The model under review builds one solid part; all positions refer to its coordinate system, in mm. Coordinates: 2 decimals unless noted, no trailing zeros. Loops run counter-clockwise (first coordinate to the right, second up) from the corner with the lowest first, then second, coordinate; pieces in that order, holes last. Notation, with made-up numbers: M -2,39 L 26,39 A21 ccw 26,55 Z; hole C 44,40.5 d4. An arc over 180 degrees is marked long. One line per item, written item: value.
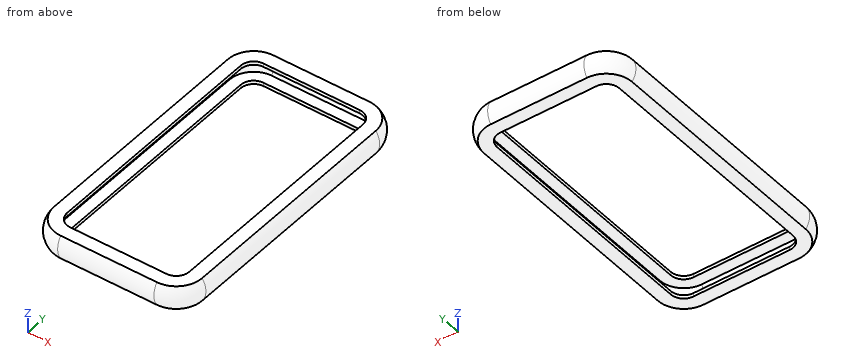
```python
from build123d import *

# Parameters (mm, degrees)
F1_DEPTH  = 5
F3_DEPTH  = 49
F5_DEPTH  = 20.5
F15_DEPTH = 1.5
F17_T     = 1.5


# Not quite as in the source:
# - a shell that OpenCascade refuses in one call is made with other operations: the cavity is built on its own and cut out


with BuildPart() as f1:
    # F0 (on Top) → F1 (new body, symmetric)
    with BuildSketch(Plane.XY):
        with BuildLine():
            Line((31.5, -49), (31.5, 49))
            ThreePointArc((31.5, 49), (28.2781745931, 56.7781745931), (20.5, 60))
            Line((20.5, 60), (-20.5, 60))
            ThreePointArc((-20.5, 60), (-28.2781745931, 56.7781745931), (-31.5, 49))
            Line((-31.5, 49), (-31.5, -49))
            ThreePointArc((-31.5, -49), (-28.2781745931, -56.7781745931), (-20.5, -60))
            Line((-20.5, -60), (20.5, -60))
            ThreePointArc((20.5, -60), (28.2781745931, -56.7781745931), (31.5, -49))
        make_face()
        with BuildLine():
            ThreePointArc((-29.5, 49), (-26.8639610307, 55.3639610307), (-20.5, 58))
            Line((-20.5, 58), (20.5, 58))
            ThreePointArc((20.5, 58), (26.8639610307, 55.3639610307), (29.5, 49))
            Line((29.5, 49), (29.5, -49))
            ThreePointArc((29.5, -49), (26.8639610307, -55.3639610307), (20.5, -58))
            Line((20.5, -58), (-20.5, -58))
            ThreePointArc((-20.5, -58), (-26.8639610307, -55.3639610307), (-29.5, -49))
            Line((-29.5, -49), (-29.5, 49))
        make_face(mode=Mode.SUBTRACT)
    extrude(amount=F1_DEPTH, both=True)

    # F2 (on Front) → F3 (join, symmetric)
    with BuildSketch(Plane.XZ):
        with BuildLine():
            Line((-31.5, -5), (-31.5, 5))
            ThreePointArc((-31.5, 5), (-33.1261364576, 0), (-31.5, -5))
        make_face()
        with BuildLine():
            ThreePointArc((31.5, -5), (33.1261364576, 0), (31.5, 5))
            Line((31.5, 5), (31.5, -5))
        make_face()
    extrude(amount=F3_DEPTH, both=True)

    # F4 (on Right) → F5 (join, symmetric)
    with BuildSketch(Plane.YZ):
        with BuildLine():
            ThreePointArc((60, -5), (61.6261364576, 0), (60, 5))
            Line((60, 5), (60, -5))
        make_face()
        with BuildLine():
            Line((-60, -5), (-60, 5))
            ThreePointArc((-60, 5), (-61.6261364576, 0), (-60, -5))
        make_face()
    extrude(amount=F5_DEPTH, both=True)

    # F7: sweep along a path in F0
    with BuildLine(Plane.XY) as f7_path:
        ThreePointArc((-20.5, 62), (-29.6923881554, 58.1923881554), (-33.5, 49))
    # F6 (on face) → F7 (sweep)
    with BuildSketch(Plane(origin=(-20.5, 0, 0), x_dir=(0, -1, 0), z_dir=(-1, 0, 0))):
        with BuildLine():
            ThreePointArc((-60, 5), (-61.6261364576, 0), (-60, -5))
            Line((-60, -5), (-60, 5))
        make_face()
    sweep(path=f7_path.line)

    # F9: sweep along a path in F0
    with BuildLine(Plane.XY) as f9_path:
        ThreePointArc((33.5, 49), (29.6923881554, 58.1923881554), (20.5, 62))
    # F8 (on face) → F9 (sweep)
    with BuildSketch(Plane.YZ.offset(20.5)):
        with BuildLine():
            Line((60, 5), (60, -5))
            ThreePointArc((60, -5), (61.6261364576, 0), (60, 5))
        make_face()
    sweep(path=f9_path.line)

    # F11: sweep along a path in F0
    with BuildLine(Plane.XY) as f11_path:
        ThreePointArc((20.5, -62), (29.6923881554, -58.1923881554), (33.5, -49))
    # F10 (on face) → F11 (sweep)
    with BuildSketch(Plane.YZ.offset(20.5)):
        with BuildLine():
            Line((-60, -5), (-60, 5))
            ThreePointArc((-60, 5), (-61.6261364576, 0), (-60, -5))
        make_face()
    sweep(path=f11_path.line)

    # F13: sweep along a path in F0
    with BuildLine(Plane.XY) as f13_path:
        ThreePointArc((-33.5, -49), (-29.6923881554, -58.1923881554), (-20.5, -62))
    # F12 (on face) → F13 (sweep)
    with BuildSketch(Plane(origin=(-20.5, 0, 0), x_dir=(0, -1, 0), z_dir=(-1, 0, 0))):
        with BuildLine():
            ThreePointArc((60, -5), (61.6261364576, 0), (60, 5))
            Line((60, 5), (60, -5))
        make_face()
    sweep(path=f13_path.line)

    # F14 (on face) → F15 (join)
    with BuildSketch(Plane.XY.offset(5)):
        with BuildLine():
            Line((20.5, 60), (-20.5, 60))
            ThreePointArc((-20.5, 60), (-28.2781745931, 56.7781745931), (-31.5, 49))
            Line((-31.5, 49), (-31.5, -49))
            ThreePointArc((-31.5, -49), (-28.2781745931, -56.7781745931), (-20.5, -60))
            Line((-20.5, -60), (20.5, -60))
            ThreePointArc((20.5, -60), (28.2781745931, -56.7781745931), (31.5, -49))
            Line((31.5, -49), (31.5, 49))
            ThreePointArc((31.5, 49), (28.2781745931, 56.7781745931), (20.5, 60))
        make_face()
        with BuildLine():
            Line((-29.5, -49), (-29.5, 49))
            ThreePointArc((-29.5, 49), (-26.8639610307, 55.3639610307), (-20.5, 58))
            Line((-20.5, 58), (20.5, 58))
            ThreePointArc((20.5, 58), (26.8639610307, 55.3639610307), (29.5, 49))
            Line((29.5, 49), (29.5, -49))
            ThreePointArc((29.5, -49), (26.8639610307, -55.3639610307), (20.5, -58))
            Line((20.5, -58), (-20.5, -58))
            ThreePointArc((-20.5, -58), (-26.8639610307, -55.3639610307), (-29.5, -49))
        make_face(mode=Mode.SUBTRACT)
        with BuildLine():
            ThreePointArc((-20.5, 58), (-26.8639610307, 55.3639610307), (-29.5, 49))
            Line((-29.5, 49), (-29.5, -49))
            ThreePointArc((-29.5, -49), (-26.8639610307, -55.3639610307), (-20.5, -58))
            Line((-20.5, -58), (20.5, -58))
            ThreePointArc((20.5, -58), (26.8639610307, -55.3639610307), (29.5, -49))
            Line((29.5, -49), (29.5, 49))
            ThreePointArc((29.5, 49), (26.8639610307, 55.3639610307), (20.5, 58))
            Line((20.5, 58), (-20.5, 58))
        make_face()
        with BuildLine():
            ThreePointArc((-26, 49), (-24.3890872965, 52.8890872965), (-20.5, 54.5))
            Line((-20.5, 54.5), (20.5, 54.5))
            ThreePointArc((20.5, 54.5), (24.3890872965, 52.8890872965), (26, 49))
            Line((26, 49), (26, -49))
            ThreePointArc((26, -49), (24.3890872965, -52.8890872965), (20.5, -54.5))
            Line((20.5, -54.5), (-20.5, -54.5))
            ThreePointArc((-20.5, -54.5), (-24.3890872965, -52.8890872965), (-26, -49))
            Line((-26, -49), (-26, 49))
        make_face(mode=Mode.SUBTRACT)
    extrude(amount=-F15_DEPTH)

    # F16: F1 across plane


with BuildPart() as f1_1:
    add(f1.part)
    add(f1.part.mirror(Plane.XY))

    # F17: shell of thickness 1.5, made by hand


with BuildPart() as f17_core1:
    # F17_t2: copy of F1
    add(f1_1.part)

    # the walls: a layer under each face that stays
    f17_faces = [f17_core1.faces().sort_by_distance(p)[0] for p in [
        (-27, -51.4285714286, -5),
        (33.1261364576, 0, 0),
        (29.4280267093, 57.9280267093, 0),
        (0, 61.6261364576, 0),
        (-29.4280267093, 57.9280267093, 0),
        (-33.1261364576, 0, 0),
        (-29.4280267093, -57.9280267093, 0),
        (0, -61.6261364576, 0),
        (29.4280267093, -57.9280267093, 0),
        (-27, -51.4285714286, 5),
        (24.3890872965, -52.8890872965, -4.25),
        (26, 0, -4.25),
        (0, -54.5, -4.25),
        (24.3890872965, 52.8890872965, -4.25),
        (-24.3890872965, -52.8890872965, -4.25),
        (0, 54.5, -4.25),
        (-26, 0, -4.25),
        (-24.3890872965, 52.8890872965, -4.25),
        (-27.5333333333, -54.1333333333, -3.5),
        (24.3890872965, -52.8890872965, 4.25),
        (26, 0, 4.25),
        (0, -54.5, 4.25),
        (24.3890872965, 52.8890872965, 4.25),
        (-24.3890872965, -52.8890872965, 4.25),
        (0, 54.5, 4.25),
        (-26, 0, 4.25),
        (-24.3890872965, 52.8890872965, 4.25),
        (-27.5333333333, -54.1333333333, 3.5),
    ]]
    thicken(f17_faces, amount=-F17_T, mode=Mode.SUBTRACT)


with BuildPart() as f1_2:
    add(f1_1.part)

    # what is left inside the walls is the cavity
    f17_cavity = [f17_core1.part.solids().sort_by_distance(p)[0] for p in [
        (-31.611136, 16.333334, 0),
    ]]
    add(f17_cavity, mode=Mode.SUBTRACT)


solid = f1_2.part
```
(1) Add section B-B on y = 39. State the section outline as (x, z) points.
Checks:
outline: M -31.5,-5 L -26,-5 L -26,-3.5 L -30.69,-3.5 A7 cw -30.69,3.5 L -26,3.5 L -26,5 L -31.5,5 A8.5 ccw Z; M 26,-5 L 31.5,-5 A8.5 ccw 31.5,5 L 26,5 L 26,3.5 L 30.69,3.5 A7 cw 30.69,-3.5 L 26,-3.5 Z
(2) Add section A-A on x = 10. State the section outline as (y, z) points.
Checks:
outline: M -60,-5 L -54.5,-5 L -54.5,-3.5 L -59.19,-3.5 A7 cw -59.19,3.5 L -54.5,3.5 L -54.5,5 L -60,5 A8.5 ccw Z; M 54.5,-5 L 60,-5 A8.5 ccw 60,5 L 54.5,5 L 54.5,3.5 L 59.19,3.5 A7 cw 59.19,-3.5 L 54.5,-3.5 Z
(3) Insertion check: pin 1 Ø1.6 at (x, z) = (-4.5, -4.5) entering from -Y; pin 2 Ø4 at (y, z) = (-37, -2.5) entering from +X; pin 3 Ø1.6 at (y, z) = (14.5, 4.5) entering from +X; pin 4 Ø5 at (x, y) = (-23, -33.5) entering from +Z. Each pin has a flat end and moves straight along its axis. Give the tip position at first contact, or say it passes through.
Checks:
pin 1: y = -60.78
pin 2: x = 33.11
pin 3: x = 32.28
pin 4: through
(4) To check wall thickness, follow L1, parallel to Z at x = -27, y = -51.5; L2, parallel to X at y = 11.5, z = -0.25; L3, parallel to Y at x = 12, z = 4.75. State the ranges of each line that lie inside material, in increasing order. Write a range as [from, to].
Checks:
L1: [-5, -3.5], [3.5, 5]
L2: [-33.12, -31.62], [31.62, 33.12]
L3: [-60.18, -54.5], [54.5, 60.18]
